Here's how the part is built. I have some questions about the finished solid (model axes, mm). A direction names the side the tool comes from. Coordinates: 2 decimals unless noted, no trailing zeros. Write each loop counter-clockwise with the first axis right and the second up, starting at its lowest first coordinate (ties: lowest second). Pieces come first, ordered by that corner, then holes.
```python
from build123d import *

# Parameters (mm, degrees)
SKETCH1_R           = 1.25
SKETCH1_R_2         = 2
SKETCH1_R_3         = 9
BOSS_EXTRUDE1_DEPTH = 3.175
SKETCH2_R           = 1.65
CUT_EXTRUDE1_DEPTH  = 164.508656116
SKETCH3_R           = 1.5
CUT_EXTRUDE2_DEPTH  = 164.508656116
SKETCH4_W           = 15
SKETCH4_H           = 15
SKETCH4_R           = 1.5
BOSS_EXTRUDE2_DEPTH = 3.175
FILLET1_DEPTH       = 3.175
FILLET1_2_DEPTH     = 3.175
FILLET2_R           = 2.5


with BuildPart() as part:
    # Sketch1 → Boss-Extrude1 (new body)
    with BuildSketch(Plane(origin=(0, 0, 0), x_dir=(1, 0, 0), z_dir=(0, 1, 0))):
        Polygon((65, -50), (10, -50), (10, 150), (-10, 150), (-10, -100), (-22.9, -100), (-22.9, -140), (-10, -140), (-10, -150), (0, -150), (10, -150), (10, -100), (65, -100), align=None)
        with Locations(Location((-18.3, -135, 0), (0, 0, 270))):
            Circle(SKETCH1_R, mode=Mode.SUBTRACT)
        with Locations(Location((-18.3, -125, 0), (0, 0, 270))):
            Circle(SKETCH1_R, mode=Mode.SUBTRACT)
        with Locations(Location((-18.3, -115, 0), (0, 0, 270))):
            Circle(SKETCH1_R, mode=Mode.SUBTRACT)
        with Locations(Location((-18.3, -105, 0), (0, 0, 270))):
            Circle(SKETCH1_R, mode=Mode.SUBTRACT)
        with Locations(Location((24, -59, 0), (0, 0, 270))):
            Circle(SKETCH1_R_2, mode=Mode.SUBTRACT)
        with Locations(Location((56, -59, 0), (0, 0, 270))):
            Circle(SKETCH1_R_2, mode=Mode.SUBTRACT)
        with Locations(Location((24, -91, 0), (0, 0, 270))):
            Circle(SKETCH1_R_2, mode=Mode.SUBTRACT)
        with Locations(Location((56, -91, 0), (0, 0, 270))):
            Circle(SKETCH1_R_2, mode=Mode.SUBTRACT)
        with Locations(Location((40, -75, 0), (0, 0, 270))):
            Circle(SKETCH1_R_3, mode=Mode.SUBTRACT)
    extrude(amount=BOSS_EXTRUDE1_DEPTH)

    # Sketch2 → Cut-Extrude1 (cut, through all)
    with BuildSketch(Plane(origin=(0, 3.175, 0), x_dir=(1, 0, 0), z_dir=(0, 1, 0))):
        with Locations(Location((40, -55, 0), (0, 0, 270))):
            Circle(SKETCH2_R)
        with Locations(Location((60, -75, 0), (0, 0, 270))):
            Circle(SKETCH2_R)
        with Locations(Location((40, -95, 0), (0, 0, 270))):
            Circle(SKETCH2_R)
        with Locations(Location((20, -75, 0), (0, 0, 270))):
            Circle(SKETCH2_R)
    extrude(amount=-CUT_EXTRUDE1_DEPTH, mode=Mode.SUBTRACT)

    # Sketch3 → Cut-Extrude2 (cut, through all)
    with BuildSketch(Plane(origin=(0, 3.175, 0), x_dir=(1, 0, 0), z_dir=(0, 1, 0))):
        with Locations(Location((0, 0, 0), (0, 0, 270))):
            Circle(SKETCH3_R)
        with Locations(Location((0, -135, 0), (0, 0, 270))):
            Circle(SKETCH3_R)
        with Locations(Location((0, 135, 0), (0, 0, 270))):
            Circle(SKETCH3_R)
    extrude(amount=-CUT_EXTRUDE2_DEPTH, mode=Mode.SUBTRACT)

    # Sketch4 → Boss-Extrude2 (add)
    # profile 1 of 5: a face of its own
    with BuildSketch(Plane(origin=(0, 3.175, 0), x_dir=(1, 0, 0), z_dir=(0, 1, 0))):
        with Locations((-17.5, 142.5)):
            Rectangle(SKETCH4_W, SKETCH4_H)
        with Locations(Location((-22.5, 137.5, 0), (0, 0, 270))):
            Circle(SKETCH4_R, mode=Mode.SUBTRACT)
        with Locations(Location((-12.5, 137.5, 0), (0, 0, 270))):
            Circle(SKETCH4_R, mode=Mode.SUBTRACT)
        with Locations(Location((-22.5, 147.5, 0), (0, 0, 270))):
            Circle(SKETCH4_R, mode=Mode.SUBTRACT)
        with Locations(Location((-12.5, 147.5, 0), (0, 0, 270))):
            Circle(SKETCH4_R, mode=Mode.SUBTRACT)
    # profile 2 of 5: a face of its own
    with BuildSketch(Plane(origin=(0, 3.175, 0), x_dir=(1, 0, 0), z_dir=(0, 1, 0))):
        with BuildLine():
            Line((17.5, 150), (10, 150))
            Line((10, 150), (10, 135))
            Line((10, 135), (17.5, 135))
            Line((17.5, 135), (17.5, 137.5))
            Line((17.5, 137.5), (14, 137.5))
            ThreePointArc((14, 137.5), (11.439339828, 136.439339828), (12.5, 139))
            Line((12.5, 139), (12.5, 146))
            ThreePointArc((12.5, 146), (11.439339828, 148.560660172), (14, 147.5))
            Line((14, 147.5), (17.5, 147.5))
            Line((17.5, 147.5), (17.5, 150))
        make_face()
    # profile 3 of 5: a face of its own
    with BuildSketch(Plane(origin=(0, 3.175, 0), x_dir=(1, 0, 0), z_dir=(0, 1, 0))):
        with BuildLine():
            Line((25, 150), (17.5, 150))
            Line((17.5, 150), (17.5, 147.5))
            Line((17.5, 147.5), (21, 147.5))
            ThreePointArc((21, 147.5), (22.5, 149), (24, 147.5))
            ThreePointArc((24, 147.5), (23.560660172, 146.439339828), (22.5, 146))
            Line((22.5, 146), (22.5, 139))
            ThreePointArc((22.5, 139), (23.560660172, 138.560660172), (24, 137.5))
            ThreePointArc((24, 137.5), (22.5, 136), (21, 137.5))
            Line((21, 137.5), (17.5, 137.5))
            Line((17.5, 137.5), (17.5, 135))
            Line((17.5, 135), (25, 135))
            Line((25, 135), (25, 150))
        make_face()
    # profile 4 of 5: a face of its own
    with BuildSketch(Plane(origin=(0, 3.175, 0), x_dir=(1, 0, 0), z_dir=(0, 1, 0))):
        with BuildLine():
            Line((21, 147.5), (17.5, 147.5))
            Line((17.5, 147.5), (17.5, 137.5))
            Line((17.5, 137.5), (21, 137.5))
            ThreePointArc((21, 137.5), (21.439339828, 138.560660172), (22.5, 139))
            Line((22.5, 139), (22.5, 146))
            ThreePointArc((22.5, 146), (21.439339828, 146.439339828), (21, 147.5))
        make_face()
    # profile 5 of 5: a face of its own
    with BuildSketch(Plane(origin=(0, 3.175, 0), x_dir=(1, 0, 0), z_dir=(0, 1, 0))):
        with BuildLine():
            Line((17.5, 137.5), (17.5, 147.5))
            Line((17.5, 147.5), (14, 147.5))
            ThreePointArc((14, 147.5), (13.560660172, 146.439339828), (12.5, 146))
            Line((12.5, 146), (12.5, 139))
            ThreePointArc((12.5, 139), (13.560660172, 138.560660172), (14, 137.5))
            Line((14, 137.5), (17.5, 137.5))
        make_face()
    extrude(amount=-BOSS_EXTRUDE2_DEPTH)

    # Fillet1: read off the stored shape, not the designer's step
    # Fillet1 outline → Fillet1 (cut)
    with BuildSketch(Plane(origin=(0, 0, 0), x_dir=(1, 0, 0), z_dir=(0, 1, 0))):
        with BuildLine():
            ThreePointArc((60, -50), (63.535533906, -51.464466094), (65, -55))
            Line((65, -55), (65, -50))
            Line((65, -50), (60, -50))
        make_face()
        with BuildLine():
            ThreePointArc((65, -95), (63.535533906, -98.535533906), (60, -100))
            Line((60, -100), (65, -100))
            Line((65, -100), (65, -95))
        make_face()
        with BuildLine():
            ThreePointArc((10, -145), (8.535533906, -148.535533906), (5, -150))
            Line((5, -150), (10, -150))
            Line((10, -150), (10, -145))
        make_face()
        with BuildLine():
            ThreePointArc((-5, -150), (-8.535533906, -148.535533906), (-10, -145))
            Line((-10, -145), (-10, -150))
            Line((-10, -150), (-5, -150))
        make_face()
        with BuildLine():
            ThreePointArc((-17.9, -140), (-21.435533906, -138.535533906), (-22.9, -135))
            Line((-22.9, -135), (-22.9, -140))
            Line((-22.9, -140), (-17.9, -140))
        make_face()
        with BuildLine():
            ThreePointArc((-22.9, -105), (-21.435533906, -101.464466094), (-17.9, -100))
            Line((-17.9, -100), (-22.9, -100))
            Line((-22.9, -100), (-22.9, -105))
        make_face()
    extrude(amount=FILLET1_DEPTH, mode=Mode.SUBTRACT)

    # Fillet1 2 outline → Fillet1 2 (add)
    with BuildSketch(Plane(origin=(0, 0, 0), x_dir=(1, 0, 0), z_dir=(0, 1, 0))):
        with BuildLine():
            Line((10, 135), (10, 130))
            ThreePointArc((10, 130), (11.464466094, 133.535533906), (15, 135))
            Line((15, 135), (10, 135))
        make_face()
        with BuildLine():
            Line((10, -50), (15, -50))
            ThreePointArc((15, -50), (11.464466094, -48.535533906), (10, -45))
            Line((10, -45), (10, -50))
        make_face()
        with BuildLine():
            Line((10, -100), (10, -105))
            ThreePointArc((10, -105), (11.464466094, -101.464466094), (15, -100))
            Line((15, -100), (10, -100))
        make_face()
        with BuildLine():
            Line((-10, -140), (-15, -140))
            ThreePointArc((-15, -140), (-11.464466094, -141.464466094), (-10, -145))
            Line((-10, -145), (-10, -140))
        make_face()
        with BuildLine():
            ThreePointArc((-15, 135), (-11.464466094, 133.535533906), (-10, 130))
            Line((-10, 130), (-10, 135))
            Line((-10, 135), (-15, 135))
        make_face()
        with BuildLine():
            ThreePointArc((-10, -95), (-11.464466094, -98.535533906), (-15, -100))
            Line((-15, -100), (-10, -100))
            Line((-10, -100), (-10, -95))
        make_face()
    extrude(amount=FILLET1_2_DEPTH)

    # Fillet2
    fillet2_edges = [part.edges().sort_by_distance(p)[0] for p in [
        (-25, 1.5875, -135),
        (-25, 1.5875, -150),
        (25, 1.5875, -150),
        (25, 1.5875, -135),
    ]]
    fillet(fillet2_edges, radius=FILLET2_R)


solid = part.part
```
1) We'd pull the mould along Z, two halves only. Please class faces 4 (the face through (63, 2, 51)), 5 (the face through (42.703, 1.565, 83.584)), 6 (the face through (-21.47, 1.57, 101.5)), 7 (the face through (64, 2, 98)): pulls with the +Z half, pulls with the -Z half, needs draft (parallel to the pull), parting line crosses it, or undercut.
Values follow:
face 4: pulls with the -Z half
face 5: undercut
face 6: undercut
face 7: pulls with the +Z half
2) On a 3-axis mill with a long thin cutter (end or side, diameter ignored), from which of +Z, -Z, +X, -X, +Y, -Y can I reach the whole of each face in a straight line? I mean faces 1 (the face through (-11, 2, 98)), 2 (the face through (-21.4, 1.57, 138.57)), 3 (the face through (11, 2, -133)). Say none if no direction works.
Values follow:
face 1: -X, +Y, -Y
face 2: +Z, -X, +Y, -Y
face 3: +X, +Y, -Y
3) Imagine slicing it at A-A on x = 34.5. Please give me the cut outline in (y, z) (3 decimals), then the cut area to 3 significant figures.
Values follow:
outline: (0, 50) - (3.175, 50) - (3.175, 67.876) - (0, 67.876) - close; (0, 82.124) - (3.175, 82.124) - (3.175, 100) - (0, 100) - close
area: 114 mm2
4) I need wall thicknesses on probe 1 along Z at (x, y) = (17, 1.35); probe 2 along X at (y, z) = (2.1, 76); probe 3 along Z at (x, y) = (54.5, 2.75). Which ranges of each line are inside material? Lowest first, please.
Values follow:
probe 1: z = -150 to -135, 50 to 100
probe 2: x = -10 to 18.69, 21.31 to 31.06, 48.94 to 58.69, 61.31 to 65
probe 3: z = 50 to 57.68, 60.32 to 89.68, 92.32 to 100
5) Imagine slicing it at B-B on z = 121. Please give me the cut outline in (x, y) (3 decimals), then the cut area to 3 significant figures.
Values follow:
outline: (-22.9, 0) - (10, 0) - (10, 3.175) - (-22.9, 3.175) - close
area: 104 mm2
6) Imagine slicing it at C-C on y = 1.9. Count the separate pieces of the cut face and the enclosed holes in it, then the cut area to 3 significant figures.
Values follow:
separate pieces: 1
enclosed holes: 24
area: 9,270 mm2
7) Imagine slicing it at D-D on z = -57.5. Please give me the cut outline in (x, y) (3 decimals), then the cut area to 3 significant figures.
Values follow:
outline: (-10, 0) - (10, 0) - (10, 3.175) - (-10, 3.175) - close
area: 63.5 mm2
8) Will these pins go through, and if not, where does the flat tip stop? pin 1 (0.9 mm diameter, centred on x = -17, y = 2, fed in from +Z); pin 2 (2 mm diameter, centred on x = -18.3, z = 105, fed in from +Y); pin 3 (1.5 mm diameter, centred on x = -11.5, y = 2.5, fed in from +Z).
Values follow:
pin 1: stops at z = 140
pin 2: passes through
pin 3: stops at z = 142.37
